```python
from build123d import *

# Parameters (mm, degrees)
F0_W     = 68
F0_H     = 5
F0_W_2   = 5
F0_H_2   = 50
F1_DEPTH = 5


with BuildPart() as f1:
    # F0 (on Front) → F1 (new body)
    with BuildSketch(Plane.XZ):
        with BuildLine():
            Line((102, -50), (170, -50))
            Line((170, -50), (170, 0))
            Line((170, 0), (170, 50))
            Line((170, 50), (5, 50))
            Line((5, 50), (5, 40))
            Line((5, 40), (0, 40))
            Line((0, 40), (0, 12.5))
            ThreePointArc((0, 12.5), (8.838835, 8.838835), (12.5, 0))
            ThreePointArc((12.5, 0), (8.838835, -8.838835), (0, -12.5))
            Line((0, -12.5), (0, -50))
            Line((0, -50), (34, -50))
            Line((34, -50), (102, -50))
        make_face()
        with Locations((68, -52.5)):
            Rectangle(F0_W, F0_H)
        with Locations((172.5, 25)):
            Rectangle(F0_W_2, F0_H_2)
        with BuildLine():
            Line((-34, -50), (0, -50))
            Line((0, -50), (0, -12.5))
            ThreePointArc((0, -12.5), (-12.5, 0), (0, 12.5))
            Line((0, 12.5), (0, 40))
            Line((0, 40), (-5, 40))
            Line((-5, 40), (-5, 50))
            Line((-5, 50), (-170, 50))
            Line((-170, 50), (-170, 0))
            Line((-170, 0), (-170, -50))
            Line((-170, -50), (-102, -50))
            Line((-102, -50), (-34, -50))
        make_face()
        with Locations((-68, -52.5)):
            Rectangle(F0_W, F0_H)
        with Locations((-172.5, 25)):
            Rectangle(F0_W_2, F0_H_2)
    extrude(amount=F1_DEPTH)


solid = f1.part
```
Here's how the part is built. I have some questions about the finished solid (model axes, mm). Round coordinates to 2 decimals unless told otherwise and drop trailing zeros. Loops run counter-clockwise (first coordinate to the right, second up) from the corner with the lowest first, then second, coordinate; pieces in that order, holes last. Notation, with made-up numbers: (38.25, 11.25) -> (54.25, 11.25) arc R27 cw to (54.25, 36.25) -> close; hole circle Ø8 at (-28, -13). An arc over 180 degrees is marked (long way). Answer as CSV lines item,"result".
1. If I drill on L1, parallel to Z at x = -15, y = -1.2; L2, parallel to X at y = -4.1, z = -43.5; L3, parallel to X at y = -4.8, z = -2, over which ranges is the centre line in solid material (lowest first)?
Final values:
L1,"z = -50 to 50"
L2,"x = -170 to 170"
L3,"x = -170 to -12.34, 12.34 to 170"
2. If we section it at C-C on x = 154: Please give me the cut outline in (y, z).
Final values:
outline,"(-5, -50) -> (0, -50) -> (0, 50) -> (-5, 50) -> close"
3. If we section it at D-D on z = -46.5: Please give me the cut outline in (x, y).
Final values:
outline,"(-170, -5) -> (170, -5) -> (170, 0) -> (-170, 0) -> close"
4. For pin 1 (2.5 mm diameter, centred on x = 8.5, y = -3.5, fed in from -Z); pin 2 (1 mm diameter, centred on y = -4, z = -17, fed in from +X); pin 3 (1.5 mm diameter, centred on y = -2, z = -51.5, fed in from +X), each with a flat end and sliding along its axis, tell me the tip position at first contact or that it passes through.
Final values:
pin 1,"stops at z = -50"
pin 2,"stops at x = 170"
pin 3,"stops at x = 102"
5. If we section it at B-B on z = 7: Please give me the cut outline in (x, y).
Final values:
outline,"(-175, -5) -> (-10.36, -5) -> (-10.36, 0) -> (-175, 0) -> close; (10.36, -5) -> (175, -5) -> (175, 0) -> (10.36, 0) -> close"
6. If we section it at A-A on y = -4.05: Please give me the cut outline in (x, z), plus the area to 3 significant figures.
Final values:
outline,"(-175, 0) -> (-170, 0) -> (-170, -50) -> (-102, -50) -> (-102, -55) -> (-34, -55) -> (-34, -50) -> (34, -50) -> (34, -55) -> (102, -55) -> (102, -50) -> (170, -50) -> (170, 0) -> (175, 0) -> (175, 50) -> (5, 50) -> (5, 40) -> (-5, 40) -> (-5, 50) -> (-175, 50) -> close; hole (0, -12.5) arc R12.5 ccw to (12.5, 0) arc R12.5 ccw (long way) to start"
area,"34,600 mm^2"
